from build123d import *

# Parameters (mm, degrees)
SKETCH1_W           = 80
SKETCH1_H           = 70
BOSS_EXTRUDE1_DEPTH = 30
SKETCH2_R           = 10
CUT_EXTRUDE1_DEPTH  = 50
FILLET1_R           = 20
FILLET2_R           = 20
FILLET3_R           = 20
FILLET4_R           = 20


with BuildPart() as part:
    # Sketch1 → Boss-Extrude1 (new body)
    with BuildSketch(Plane(origin=(0, 0, 0), x_dir=(0, 0, -1), z_dir=(1, 0, 0))):
        Rectangle(SKETCH1_W, SKETCH1_H)
    extrude(amount=BOSS_EXTRUDE1_DEPTH)

    # Sketch2 → Cut-Extrude1 (cut)
    with BuildSketch(Plane.XY.offset(40)):
        with Locations((15, 0)):
            Circle(SKETCH2_R)
    extrude(amount=-CUT_EXTRUDE1_DEPTH, mode=Mode.SUBTRACT)

    # Fillet1
    fillet1_edges = [part.edges().sort_by_distance(p)[0] for p in [
        (15, 35, -40),
    ]]
    fillet(fillet1_edges, radius=FILLET1_R)

    # Fillet2
    fillet2_edges = [part.edges().sort_by_distance(p)[0] for p in [
        (15, -35, -40),
    ]]
    fillet(fillet2_edges, radius=FILLET2_R)

    # Fillet3
    fillet3_edges = [part.edges().sort_by_distance(p)[0] for p in [
        (15, -35, 40),
    ]]
    fillet(fillet3_edges, radius=FILLET3_R)

    # Fillet4
    fillet4_edges = [part.edges().sort_by_distance(p)[0] for p in [
        (15, 35, 40),
    ]]
    fillet(fillet4_edges, radius=FILLET4_R)


solid = part.part
The model under review builds one solid part; all positions refer to its coordinate system, in mm. A direction names the side the tool comes from. Round coordinates to 2 decimals unless told otherwise and drop trailing zeros. Write each loop counter-clockwise with the first axis right and the second up, starting at its lowest first coordinate (ties: lowest second). Pieces come first, ordered by that corner, then holes. Notation, with made-up numbers: (73.25, 7.25) - (100.25, 7.25) arc R7 ccw to (100.25, 12.25) - close; hole circle Ø5 at (-32.5, 54.5). An arc over 180 degrees is marked (long way). One line per item, written item: value. Start each with the question number.
1. Consider section D-D on x = 2. Write out the cut boundary in (y, z), and give its area (3 significant figures).
2. To check wall thickness, follow L1, parallel to Y at x = 15, z = 11; L2, parallel to Y at x = 22, z = 9.5; L3, parallel to X at y = -8, z = 8. State the ranges of each line that lie inside material, in increasing order. Write a range as from..to.
3. Consider section B-B on y = 0. Write out the cut boundary in (x, z), and give its area (3 significant figures).
4. Machinability: for faces 1 (the face through (15, 0, -10)), 2 (the face through (15.21, 29.297, -33.986)), which of the approach directions +Z, -Z, +X, -X, +Y, -Y give a long, thin tool a straight path to every point of the face, cutting with its end or side? Answer none if there is none.
5. The part is to be moulded in two halves that separate along X. For faces 3 (the face through (15.21, 28.986, 34.297)), 4 (the face through (24.54, 3, 15.35)), 5 (the face through (30, 0, 1)), say which applies: released by +X, released by -X, zero draft, split by the parting line, or undercut.
6. Clearance check with flat-ended pins moving along their axes: P1, Ø8, axis at x = 7, z = 30.5, coming from the +Y side; P2, Ø6, axis at x = 15, y = 2.5, coming from the +Z side. State where each tip first meets the part, or that it passes through.
7. Consider section C-C on x = 15. Write out the cut boundary in (y, z).
8. Consider section A-A on z = -5. Write out the cut boundary in (x, y), and give its area (3 significant figures).
Checks:
1. outline: (-35, -20) arc R20 ccw to (-15, -40) - (15, -40) arc R20 ccw to (35, -20) - (35, 20) arc R20 ccw to (15, 40) - (-15, 40) arc R20 ccw to (-35, 20) - close
1. area: 5,260 mm^2
2. L1: y = -35..-10, 10..35
2. L2: y = -35..-7.14, 7.14..35
2. L3: x = 0..9, 21..30
3. outline: (0, -40) - (30, -40) - (30, 40) - (25, 40) - (25, -10) - (5, -10) - (5, 40) - (0, 40) - close
3. area: 1,400 mm^2
4. face 1: +Z
4. face 2: -Z, +X, -X, +Y
5. face 3: zero draft
5. face 4: undercut
5. face 5: released by +X
6. P1: stops at y = 33.91
6. P2: stops at z = -10
7. outline: (-35, -20) arc R20 ccw to (-15, -40) - (15, -40) arc R20 ccw to (35, -20) - (35, 20) arc R20 ccw to (15, 40) - (10, 40) - (10, -10) - (-10, -10) - (-10, 40) - (-15, 40) arc R20 ccw to (-35, 20) - close
8. outline: (0, -35) - (30, -35) - (30, 35) - (0, 35) - close; hole circle Ø20 at (15, 0)
8. area: 1,790 mm^2
